Build history of the part. All positions in model axes, mm. Coordinates: 2 decimals unless noted, no trailing zeros. Loops run counter-clockwise (first coordinate to the right, second up) from the corner with the lowest first, then second, coordinate; pieces in that order, holes last.
(1) Two-plate mould, pull along Y, no slides. Class faces 1 (the face through (25.4, 1, -1)), 2 (the face through (13.66, 0.48, -0.63)), 3 (the face through (14.561, 1.468, -1.915)): pulls with the +Y half, pulls with the -Y half, needs draft (parallel to the pull), parting line crosses it, or undercut.
(2) Slice it at A-A (z = 0). Give the cut face in (x, y) (1 decimal), and give its area (3 significant figures).
(3) Flat gauge pins, fed straight in: P1, Ø0.5, axis at y = 0, z = 0.5, coming from the +X side; P2, Ø2, axis at x = 11, y = 2, coming from the -Z side; P3, Ø1.5, axis at x = 3.5, z = 1, coming from the -Y side. Where does each tip first touch, or does it go through?
(4) Slice it at C-C (x = 3.25). Give the cut face in (y, z) (1 decimal), and give its area (3 significant figures).
(5) Slice it at B-B (x = 7). Give the cut face in (y, z), and give its area (3 significant figures).
(6) Wall check: L1, parallel to Y at x = 12.75, z = 0; L2, parallel to X at y = 2.25, z = -0.5; L3, parallel to Y at x = 0.55, z = 0. Give the ranges that are in metal, low to high.
from build123d import *


with BuildPart() as part:
    # Sketch1 → Revolve1 (revolve)
    with BuildSketch(Plane.XY, mode=Mode.PRIVATE) as revolve1_sk:
        with BuildLine():
            Line((0, 0.3556), (1.5875, 0.3556))
            Line((1.5875, 0.3556), (1.5875, 0.79375))
            Line((1.5875, 0.79375), (25.4, 0.79375))
            Line((25.4, 0.79375), (25.4, 2.413))
            Line((25.4, 2.413), (25.4, 3.175))
            ThreePointArc((25.4, 3.175), (25.176815367, 2.636184633), (24.638, 2.413))
            Line((24.638, 2.413), (4.7625, 2.413))
            Line((4.7625, 2.413), (4.7625, 1.5875))
            Line((4.7625, 1.5875), (2.974069687, 1.5875))
            Line((2.974069687, 1.5875), (0, 0.3556))
        make_face()
    revolve(revolve1_sk.sketch.rotate(Axis((0, 0, 0), (1, 0, 0)), 90), axis=Axis((0, 0, 0), (1, 0, 0)))


solid = part.part
Response values:
1. face 1: needs draft
1. face 2: undercut
1. face 3: parting line crosses it
2. outline: (0, -0.4) - (3, -1.6) - (4.8, -1.6) - (4.8, -2.4) - (24.6, -2.4) arc R0.8 cw to (25.4, -3.2) - (25.4, -0.8) - (1.6, -0.8) - (1.6, -0.4) - close; (0, 0.4) - (1.6, 0.4) - (1.6, 0.8) - (25.4, 0.8) - (25.4, 3.2) arc R0.8 cw to (24.6, 2.4) - (4.8, 2.4) - (4.8, 1.6) - (3, 1.6) - close
2. area: 72.4 mm2
3. P1: stops at x = 1.59
3. P2: stops at z = -2.2
3. P3: stops at y = -1.57
4. outline: circle Ø3.2 at (0, 0); hole circle Ø1.6 at (0, 0)
4. area: 5.94 mm2
5. outline: circle Ø4.83 at (0, 0); hole circle Ø1.59 at (0, 0)
5. area: 16.3 mm2
6. L1: y = -2.41 to -0.79, 0.79 to 2.41
6. L2: x = 4.76 to 25.4
6. L3: y = -0.58 to -0.36, 0.36 to 0.58
